Work out the finished part from the listing and answer in its coordinate system (mm). Face numbers are marked on the shaded views. A direction names the side the tool comes from. Give positions to 0.01 mm unless a question says otherwise; leave off trailing zeros. Write each loop counter-clockwise with the first axis right and the second up, starting at its lowest first coordinate (ties: lowest second). Pieces come first, ordered by that corner, then holes.
1) Find section A-A (y = 0). Determine the outline of the cut face in (x, z), plus the area to 3 significant figures.
2) Find section B-B (z = 2.75). Determine the outline of the cut face in (x, y), plus the area to 3 significant figures.
3) Determine the mould class of the marked faces 1, 2 and 3 for opening direction Y: pulls with the +Y half, pulls with the -Y half, needs draft (parallel to the pull), parting line crosses it, or undercut.
4) Given pin 1 Ø1 at (y, z) = (-3.5, 10) entering from +X; pin 2 Ø3 at (y, z) = (-2, 9) entering from -X; pin 3 Ø2 at (x, z) = (2.5, 6.5) entering from +Y, each flat-ended and moving along its own axis, determine where each tip first touches the part or whether it passes through.
5) Straight lines are drawn through the part: probe 1 along Y at (x, z) = (0, 5.75); probe 2 along Y at (x, z) = (0, 9.15); probe 3 along X at (y, z) = (-1.5, 9). For each, find the intervals that lie inside material, in ascending order.
6) A tool of negligible diameter and unlimited length cuts with its end or side. For the marked faces 4 and 5, from which of +Z, -Z, +X, -X, +Y, -Y can it reach the whole face along a straight path? Write none if from no direction.
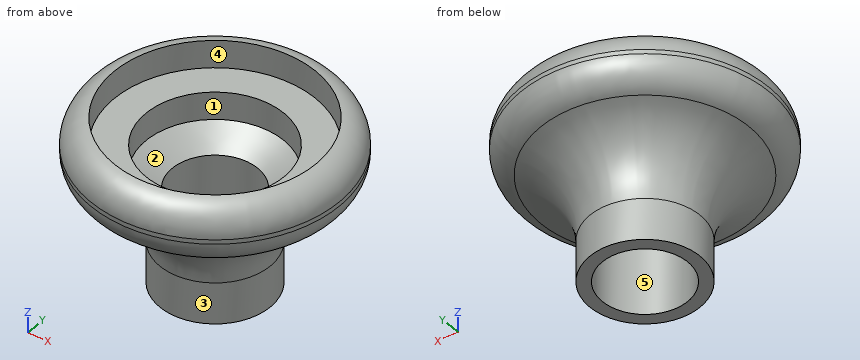
```python
from build123d import *


with BuildPart() as f1:
    # F0 (on Front) → F1 (revolve)
    with BuildSketch(Plane.XZ):
        with BuildLine():
            Line((9, 9.708204), (9, 10.022628))
            ThreePointArc((9, 10.022628), (8.516575, 11.326468), (7.3, 12))
            Line((7.3, 12), (7.3, 10))
            Line((7.3, 10), (5, 10))
            Line((5, 10), (5, 8))
            Line((5, 8), (3.1, 6.858365))
            Line((3.1, 6.858365), (3.1, 0))
            Line((3.1, 0), (4, 0))
            Line((4, 0), (4, 3))
            ThreePointArc((4, 3), (4.991081, 5.988072), (7.571429, 7.791574))
            ThreePointArc((7.571429, 7.791574), (8.603567, 8.512975), (9, 9.708204))
        make_face()
    revolve(axis=Axis((0, 0, 6), (0, 0, 1)))


solid = f1.part
```
Results:
1. outline: (-9, 9.71) arc R2 ccw to (-7.57, 7.79) arc R5 cw to (-4, 3) - (-4, 0) - (-3.1, 0) - (-3.1, 6.86) - (-5, 8) - (-5, 10) - (-7.3, 10) - (-7.3, 12) arc R2 ccw to (-9, 10.02) - close; (3.1, 0) - (4, 0) - (4, 3) arc R5 cw to (7.57, 7.79) arc R2 ccw to (9, 9.71) - (9, 10.02) arc R2 ccw to (7.3, 12) - (7.3, 10) - (5, 10) - (5, 8) - (3.1, 6.86) - close
1. area: 43.1 mm2
2. outline: circle Ø8 at (0, 0); hole circle Ø6.2 at (0, 0)
2. area: 20.1 mm2
3. face 1: undercut
3. face 2: undercut
3. face 3: parting line crosses it
4. pin 1: stops at x = 8.49
4. pin 2: stops at x = -8.98
4. pin 3: stops at y = 6.38
5. probe 1: y = -4.82 to -3.1, 3.1 to 4.82
5. probe 2: y = -8.92 to -5, 5 to 8.92
5. probe 3: x = -8.74 to -4.77, 4.77 to 8.74
6. face 4: +Z
6. face 5: +Z, -Z
